For this review, take the finished solid that the model builds, in its own axes (mm). A direction names the side the tool comes from. Round coordinates to 2 decimals unless told otherwise and drop trailing zeros. Order: outer loops, then holes, each group sorted by start corner. A loop starts at its lowest first (then second) coordinate and runs counter-clockwise, first axis right, second up. Notation, with made-up numbers: M 35.25,13.25 L 80.25,13.25 A30 ccw 80.25,38.25 Z; hole C -35,9.5 d2. An arc over 180 degrees is marked long. Put each result on its own line as item: value.
from build123d import *

# Parameters (mm, degrees)
F1_DEPTH        = 35
F2_DEPTH        = 35
F6_D            = 3.5
F6_DEPTH        = 12
F6_CBORE_D      = 6.5
F6_CBORE_DEPTH  = 2.5
F6_TIP          = 1.0515060833
F7_D            = 3.5
F7_DEPTH        = 12
F7_CBORE_D      = 6.5
F7_CBORE_DEPTH  = 2.5
F7_TIP          = 1.0515060833
F8_D            = 3.5
F8_DEPTH        = 12
F8_CBORE_D      = 6.5
F8_CBORE_DEPTH  = 2.5
F8_TIP          = 1.0515060833
F3_R            = 2.5
F9_DEPTH        = 25
F11_D           = 6.5
F11_DEPTH       = 35
F11_CBORE_D     = 10
F11_CBORE_DEPTH = 25
F11_TIP         = 1.9527970118


with BuildPart() as f1:
    # F0 (on Top) → F1 (new body)
    with BuildSketch(Plane.XY):
        with BuildLine():
            Line((-2.5, 7.5993420768), (-2.5, 1.443375673))
            Line((-2.5, 1.443375673), (2.5, 1.443375673))
            Line((2.5, 1.443375673), (2.5, 7.5993420768))
            ThreePointArc((2.5, 7.5993420768), (0, 8), (-2.5, 7.5993420768))
        make_face()
        with BuildLine():
            Line((-2.5, 53.443375673), (-2.5, 7.5993420768))
            ThreePointArc((-2.5, 7.5993420768), (0, 8), (2.5, 7.5993420768))
            Line((2.5, 7.5993420768), (2.5, 53.443375673))
            Line((2.5, 53.443375673), (-2.5, 53.443375673))
        make_face()
        with BuildLine():
            Line((7.8312232905, -1.6346075289), (2.5, 1.443375673))
            Line((2.5, 1.443375673), (0, -2.8867513459))
            Line((0, -2.8867513459), (5.3312232905, -5.9647345479))
            ThreePointArc((5.3312232905, -5.9647345479), (6.9282032303, -4), (7.8312232905, -1.6346075289))
        make_face()
        Polygon((2.5, 1.443375673), (-2.5, 1.443375673), (0, -2.8867513459), align=None)
        with BuildLine():
            Line((0, -2.8867513459), (-2.5, 1.443375673))
            Line((-2.5, 1.443375673), (-7.8312232905, -1.6346075289))
            ThreePointArc((-7.8312232905, -1.6346075289), (-6.9282032303, -4), (-5.3312232905, -5.9647345479))
            Line((-5.3312232905, -5.9647345479), (0, -2.8867513459))
        make_face()
        with BuildLine():
            Line((47.5333209968, -24.556624327), (7.8312232905, -1.6346075289))
            ThreePointArc((7.8312232905, -1.6346075289), (6.9282032303, -4), (5.3312232905, -5.9647345479))
            Line((5.3312232905, -5.9647345479), (45.0333209968, -28.8867513459))
            Line((45.0333209968, -28.8867513459), (47.5333209968, -24.556624327))
        make_face()
        with BuildLine():
            ThreePointArc((-5.3312232905, -5.9647345479), (-6.9282032303, -4), (-7.8312232905, -1.6346075289))
            Line((-7.8312232905, -1.6346075289), (-47.5333209968, -24.556624327))
            Line((-47.5333209968, -24.556624327), (-45.0333209968, -28.8867513459))
            Line((-45.0333209968, -28.8867513459), (-5.3312232905, -5.9647345479))
        make_face()
    extrude(amount=F1_DEPTH)

    # F0 (on Top) → F2 (join)
    with BuildSketch(Plane.XY):
        with BuildLine():
            Line((-7.8312232905, -1.6346075289), (-2.5, 1.443375673))
            Line((-2.5, 1.443375673), (-2.5, 7.5993420768))
            ThreePointArc((-2.5, 7.5993420768), (-6.9282032303, 4), (-7.8312232905, -1.6346075289))
        make_face()
        with BuildLine():
            Line((2.5, 7.5993420768), (2.5, 1.443375673))
            Line((2.5, 1.443375673), (7.8312232905, -1.6346075289))
            ThreePointArc((7.8312232905, -1.6346075289), (7.9576939601, -0.8216488531), (8, 0))
            ThreePointArc((8, 0), (6.4807406984, 4.6904157598), (2.5, 7.5993420768))
        make_face()
        with BuildLine():
            Line((5.3312232905, -5.9647345479), (0, -2.8867513459))
            Line((0, -2.8867513459), (-5.3312232905, -5.9647345479))
            ThreePointArc((-5.3312232905, -5.9647345479), (0, -8), (5.3312232905, -5.9647345479))
        make_face()
    extrude(amount=F2_DEPTH)

    # F6
    with Locations(Plane(origin=(-1.25, -2.1650635095, 0), x_dir=(0.8660254038, -0.5, 0), z_dir=(-0.5, -0.8660254038, 0))):
        with Locations((25.443375673, 29.5), (45.443375673, 29.5), (35.443375673, 6)):
            CounterBoreHole(F6_D / 2, F6_CBORE_D / 2, F6_CBORE_DEPTH, depth=F6_DEPTH)
            with Locations((0, 0, -(F6_DEPTH + F6_TIP / 2))):  # 118° drill point
                Cone(0, F6_D / 2, F6_TIP, mode=Mode.SUBTRACT)

    # F7
    with Locations(Plane.YZ.offset(2.5)):
        with Locations((25.443375673, 29.5), (45.443375673, 29.5), (35.443375673, 6)):
            CounterBoreHole(F7_D / 2, F7_CBORE_D / 2, F7_CBORE_DEPTH, depth=F7_DEPTH)
            with Locations((0, 0, -(F7_DEPTH + F7_TIP / 2))):  # 118° drill point
                Cone(0, F7_D / 2, F7_TIP, mode=Mode.SUBTRACT)

    # F8
    with Locations(Plane(origin=(-1.25, 2.1650635095, 0), x_dir=(-0.8660254038, -0.5, 0), z_dir=(-0.5, 0.8660254038, 0))):
        with Locations((25.443375673, 29.5), (45.443375673, 29.5), (35.443375673, 6)):
            CounterBoreHole(F8_D / 2, F8_CBORE_D / 2, F8_CBORE_DEPTH, depth=F8_DEPTH)
            with Locations((0, 0, -(F8_DEPTH + F8_TIP / 2))):  # 118° drill point
                Cone(0, F8_D / 2, F8_TIP, mode=Mode.SUBTRACT)

    # F3 (on face) → F9 (cut)
    with BuildSketch(Plane(origin=(-1.25, -2.1650635095, 0), x_dir=(0.8660254038, -0.5, 0), z_dir=(-0.5, -0.8660254038, 0))):
        with Locations((13.5993420768, 6)):
            Circle(F3_R)
    extrude(amount=-F9_DEPTH, mode=Mode.SUBTRACT)

    # F11
    with Locations(Plane.XY.offset(35)):
        with Locations((0, 0)):
            CounterBoreHole(F11_D / 2, F11_CBORE_D / 2, F11_CBORE_DEPTH, depth=F11_DEPTH)
            with Locations((0, 0, -(F11_DEPTH + F11_TIP / 2))):  # 118° drill point
                Cone(0, F11_D / 2, F11_TIP, mode=Mode.SUBTRACT)


solid = f1.part
(1) To check wall thickness, follow L1, parallel to Y at x = 0, z = 21.75; L2, parallel to X at y = 9, z = 2; L3, parallel to X at y = -13.5, z = 11. State the ranges of each line that lie inside material, in increasing order.
A:
L1: y = -8 to -5, 5 to 53.44
L2: x = -2.5 to 2.5
L3: x = -28.38 to -18.38, 18.38 to 28.38
(2) Add section A-A on z = 14.5. Give the boundary of the cut face in (x, y).
A:
outline: M -47.53,-24.56 L -45.03,-28.89 L -5.33,-5.96 A8 ccw 5.33,-5.96 L 45.03,-28.89 L 47.53,-24.56 L 7.83,-1.63 A8 ccw 2.5,7.6 L 2.5,53.44 L -2.5,53.44 L -2.5,7.6 A8 ccw -7.83,-1.63 Z; hole C 0,0 d10
(3) For faces 4 (the face through (-25.46, -17.586, 17.255)), 5 (the face through (1.268, 26.943, 26.617)), 6 (the face through (-1.08, -4.88, 22.68)), list the 3-axis set-ups (+Z, -Z, +X, -X, +Y, -Y) from which the entire face can be reached by the end or side of a thin tool; tool diameter is ignored.
A:
face 4: +Z, -Z, -Y
face 5: +X
face 6: +Z
(4) Insertion check: pin 1 Ø1.5 at (x, y) = (0, 6.5) entering from -Z; pin 2 Ø3 at (y, z) = (46, 29) entering from +X; pin 3 Ø2 at (y, z) = (-17.5, 9) entering from -X; pin 4 Ø5 at (y, z) = (45.44, 29.5) entering from -X. Each pin has a flat end and moves straight along its axis. Give the tip position at first contact, or say it passes through.
A:
pin 1: stops at z = 0
pin 2: stops at x = 0
pin 3: stops at x = -37.04
pin 4: stops at x = -2.5
(5) Add section C-C on y = 30.5. Give the boundary of the cut face in (x, z), then the cut area to 3 significant figures.
A:
outline: M -2.5,0 L 2.5,0 L 2.5,35 L -2.5,35 Z
area: 175 mm2
(6) Add section B-B on z = 29.5. State how many separate pieces and enclosed holes the cut face has, then the cut area to 3 significant figures.
A:
separate pieces: 7
enclosed holes: 1
area: 656 mm2
(7) Draft analysis for pull direction Y (two halves, no side actions). For faces 1 (the face through (0, -6, 35)), 2 (the face through (46.266, -26.752, 17.255)), 3 (the face through (-23.246, -13.421, 28.101)), state which applies: released by +Y, released by -Y, zero draft, split by the parting line, or undercut.
A:
face 1: zero draft
face 2: released by -Y
face 3: undercut
